The figure shows three views and two pictorial views of one solid part (mm, origin at its lowest corner). Answer the questions. Give positions to 0.01 mm unless a question says otherwise; leave off trailing zeros. Loops run counter-clockwise (first coordinate to the right, second up) from the corner with the lowest first, then second, coordinate; pieces in that order, holes last. Notation, with made-up numbers: (2, -26) - (7, -26) arc R28 cw to (7, -1) - close; hole circle Ø9 at (65, 27). An arc over 180 degrees is marked (long way). Use a Markdown table: item, result. Add a question column.
Item 1: A cutting plane is placed at D-D (x = 14). Determine the outline of the cut face in (y, z), plus the area to 3 significant figures.
Item 2: A cutting plane is placed at C-C (y = 3). Determine the outline of the cut face in (x, z).
Item 3: A cutting plane is placed at B-B (x = 10.5). Determine the outline of the cut face in (y, z), plus the area to 3 significant figures.
Item 4: Consider probe 1 along Y at (x, z) = (10.5, 3); probe 2 along Y at (x, z) = (10, 2); probe 3 along Y at (x, z) = (11.5, 0.75). Determine where each line is inside the solid, lowest interval first. Write a range as [from, to].
Item 5: For a pull along Y with two mould halves and no side action, classify the marked faces 1, 2, 3 and 4 as +Y half, -Y half, draft (parallel to the pull), parting line (faces both ways), or undercut.
Item 6: A cutting plane is placed at A-A (z = 4). Determine the outline of the cut face in (x, y), plus the area to 3 significant figures.
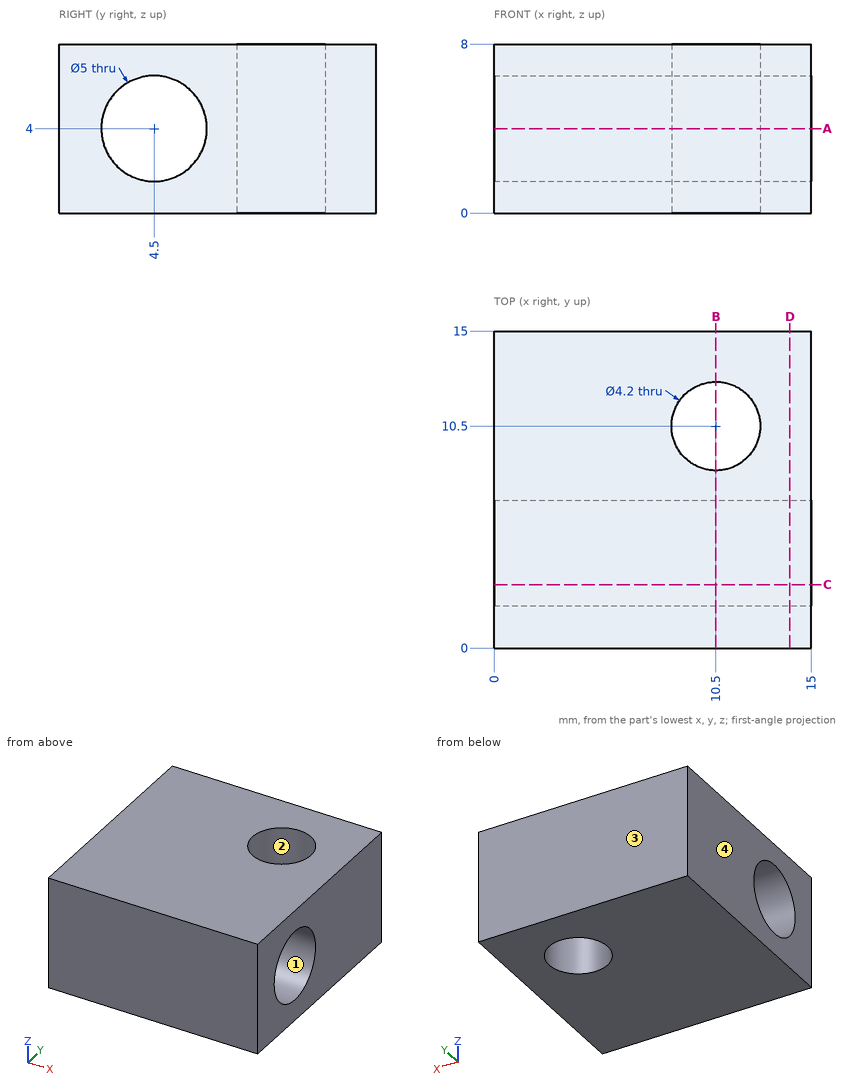
Geometry says:
| question | item | result |
|---|---|---|
| 1 | outline | (0, 0) - (15, 0) - (15, 8) - (0, 8) - close; hole circle Ø5 at (4.5, 4) |
| 1 | area | 100 mm² |
| 2 | outline | (0, 0) - (15, 0) - (15, 2) - (0, 2) - close; (0, 6) - (15, 6) - (15, 8) - (0, 8) - close |
| 3 | outline | (0, 0) - (8.4, 0) - (8.4, 8) - (0, 8) - close; (12.6, 0) - (15, 0) - (15, 8) - (12.6, 8) - close; hole circle Ø5 at (4.5, 4) |
| 3 | area | 66.8 mm² |
| 4 | probe 1 | [0, 2.21], [6.79, 8.4], [12.6, 15] |
| 4 | probe 2 | [0, 3], [6, 8.46], [12.54, 15] |
| 4 | probe 3 | [0, 8.65], [12.35, 15] |
| 5 | face 1 | undercut |
| 5 | face 2 | undercut |
| 5 | face 3 | +Y half |
| 5 | face 4 | draft |
| 6 | outline | (0, 0) - (15, 0) - (15, 2) - (0, 2) - close; (0, 7) - (15, 7) - (15, 15) - (0, 15) - close; hole circle Ø4.2 at (10.5, 10.5) |
| 6 | area | 136 mm² |
